Autodesk Inventor part; units mm, degrees
ref_plane "YZ Plane" through (0, 0, 0) normal (1, 0, 0) x (0, 1, 0)
ref_plane "XZ Plane" through (0, 0, 0) normal (0, 1, 0) x (-1, 0, 0)
ref_plane "XY Plane" through (0, 0, 0) normal (0, 0, 1) x (1, 0, 0)
ref_plane "Work Plane5" through (0, 3, 0) normal (0, 1, 0) x (1, 0, 0)
sketch "Sketch45" plane through (0, 3, 0) normal (0, 1, 0) x (1, 0, 0)
  line L0 (35, -20) -> (-3, -20)
  line L1 (-3, -20) -> (-3, 20)
  line L2 (-3, 20) -> (35, 20)
  line L3 (35, 20) -> (35, -20)
  point P0 (0, 0)
  dimension "d142" = 38
  dimension "d143" = 40
extrude "Extrusion34" add sketch "Sketch45" along normal blind 30
ref_plane "Work Plane2" through (0, 0, 0) normal (0, -1, 0) x (1, 0, 0)
sketch "Sketch47" plane through (0, 0, 0) normal (0, -1, 0) x (1, 0, 0)
  circle A0 centre (16, 0) radius 18
  point P0 (0, 0)
  dimension "d146" = 36
extrude "Extrusion35" cut sketch "Sketch47" against normal blind 30 draft -15
ref_plane "Work Plane1" through (0, 3, 0) normal (0, 1, 0) x (1, 0, 0)
sketch "Sketch74" plane through (0, 33, 0) normal (0, 1, 0) x (1, 0, 0)
  circle A0 centre (20, 0) radius 1.15
  point P0 (0, 0)
  dimension "d210" = 2.3
extrude "Extrusion51" cut sketch "Sketch74" against normal blind 10
sketch "Sketch77" plane through (0, 3, 0) normal (0, -1, 0) x (1, 0, 0)
  circle A0 centre (16, 0) radius 17.5
  point P0 (0, 0)
  dimension "d219" = 35
sketch "Sketch78" plane through (0, 3, 0) normal (0, -1, 0) x (1, 0, 0)
  line L0 (45, -30) -> (-13, -30)
  line L1 (-13, -30) -> (-13, 30)
  line L2 (-13, 30) -> (45, 30)
  line L3 (45, 30) -> (45, -30)
  line L4 (45, -30) -> (-13, 30) construction
  line L5 (-13, -30) -> (45, 30) construction
  point P0 (0, 0)
  point P1 (16, 0)
  dimension "d220" = 58
  dimension "d221" = 60
extrude "Extrusion53" add sketch "Sketch78" against normal blind 3
extrude "Extrusion54" cut sketch "Sketch77" against normal blind 3
sketch "Sketch81" plane through (0, 3, 0) normal (0, -1, 0) x (1, 0, 0)
  circle A0 centre (33.5, -25) radius 2.7
  line L0 (-13, -30) -> (45, -30)
  line L1 (45, -30) -> (45, 30)
  circle A1 centre (16, -25) radius 2.7
  circle A2 centre (-1.5, -25) radius 2.7
  circle A3 centre (-1.5, 25) radius 2.7
  circle A4 centre (16, 25) radius 2.7
  circle A5 centre (33.5, 25) radius 2.7
  point P0 (0, 0)
  dimension "mag_D" = 5.4
  dimension "d232" = 5
  dimension "d233" = 11.5
  dimension "d234" = 5.4
  dimension "d235" = 17.5
  dimension "d236" = 5.4
  dimension "d237" = 17.5
  dimension "d243" = 5.4
  dimension "d245" = 5.4
  dimension "d246" = 17.5
  dimension "d247" = 5.4
  dimension "d248" = 17.5
extrude "Extrusion56" cut sketch "Sketch81" against normal blind 30
equation "\"d234\" = mag_D"
equation "\"d236\" = mag_D"
equation "\"d237\" = d235"
equation "\"d243\" = mag_D"
equation "\"d245\" = mag_D"
equation "\"d246\" = d235"
equation "\"d247\" = mag_D"
equation "\"d248\" = d235"
properties part number "liquid_port_v06"
Read the model definition and answer for the solid it produces. Units are mm, in the model's axes. A direction names the side the tool comes from. Coordinates: 2 decimals unless noted, no trailing zeros. Loops run counter-clockwise (first coordinate to the right, second up) from the corner with the lowest first, then second, coordinate; pieces in that order, holes last.
(1) A tool of negligible diameter and unlimited length cuts with its end or side. For faces 5 (the face through (16, 19, 20)), 6 (the face through (2.113, 4.479, -10.648)), 7 (the face through (35, 19, 0)), 8 (the face through (-3, 19, 0)), from which of +Z, -Z, +X, -X, +Y, -Y can it reach the whole face along a straight path? Write none if from no direction.
Solution:
face 5: +Z, +X, -X, +Y
face 6: -Y
face 7: +Z, -Z, +X, +Y
face 8: +Z, -Z, -X, +Y
(2) The part is cut by section D-D (y = 9). Determine the outline of the cut face in (x, z).
Solution:
outline: (-3, -20) - (35, -20) - (35, 20) - (-3, 20) - close; hole circle Ø31.18 at (16, 0)
(3) The part is cut by section C-C (z = -19). Determine the outline of the cut face in (x, y).
Solution:
outline: (-13, 3) - (45, 3) - (45, 6) - (35, 6) - (35, 33) - (-3, 33) - (-3, 6) - (-13, 6) - close
(4) The part is cut by section B-B (z = 0). Determine the outline of the cut face in (x, y).
Solution:
outline: (-13, 3) - (-1.5, 3) - (-1.5, 6) - (-0.39, 6) - (6.04, 30) - (18.85, 30) - (18.85, 33) - (-3, 33) - (-3, 6) - (-13, 6) - close; (21.15, 30) - (25.96, 30) - (32.39, 6) - (33.5, 6) - (33.5, 3) - (45, 3) - (45, 6) - (35, 6) - (35, 33) - (21.15, 33) - close
(5) Consider line 1 along X through (y, z) = (30.8, 0); line 2 along Z through (x, y) = (20, 32.4); line 3 along Y through (x, z) = (17, 7.5). Determine where each line is inside the solid, lowest interval first.
Solution:
line 1: x = -3 to 18.85, 21.15 to 35
line 2: z = -20 to -1.15, 1.15 to 20
line 3: y = 30 to 33
(6) Flat-ended cylindrical pins translate along their axes: pin 1 Ø10 at (x, y) = (-2.5, 11.5) entering from +Z; pin 2 Ø6 at (x, y) = (11, 24) entering from -Z; pin 3 Ø4 at (y, z) = (9, -7) entering from +X. Find the tip coordinate at first contact, or state that the pin passes through.
Solution:
pin 1: stops at z = 20
pin 2: stops at z = -20
pin 3: stops at x = 35
(7) The part is cut by section A-A (x = 16). Determine the outline of the cut face in (y, z).
Solution:
outline: (3, -30) - (6, -30) - (6, -27.7) - (3, -27.7) - close; (3, -22.3) - (6, -22.3) - (6, -20) - (33, -20) - (33, 20) - (6, 20) - (6, 22.3) - (3, 22.3) - (3, 17.5) - (6, 17.5) - (6, 16.39) - (30, 9.96) - (30, -9.96) - (6, -16.39) - (6, -17.5) - (3, -17.5) - close; (3, 27.7) - (6, 27.7) - (6, 30) - (3, 30) - close
(8) The mould has two halves that part along Z. Classify faces 1 (the face through (21, 6, 16)), 2 (the face through (-13, 4, 0)), 3 (the face through (17.452, 4.479, -22.723)), 4 (the face through (16, 19, -20)): released by +Z, released by -Z, zero draft, split by the parting line, or undercut.
Solution:
face 1: undercut
face 2: zero draft
face 3: undercut
face 4: released by -Z
